Input: part model. Units: mm. Frame: model coordinates. A direction names the side the tool comes from. Round coordinates to 2 decimals unless told otherwise and drop trailing zeros. Write each loop counter-clockwise with the first axis right and the second up, starting at its lowest first coordinate (ties: lowest second). Pieces come first, ordered by that corner, then holes. Notation, with made-up numbers: (-9.75, 42.25) - (-3.75, 42.25) arc R38 ccw to (-3.75, 81.25) - close; hole circle Ø1 at (57, -30.5). An arc over 180 degrees is marked (long way). Use one line per item in the form item = value.
```python
from build123d import *

# Parameters (mm, degrees)
SKETCH1_R           = 2.25
SKETCH1_R_2         = 1.5
BOSS_EXTRUDE1_DEPTH = 1


with BuildPart() as part:
    # Sketch1 → Boss-Extrude1 (new body)
    with BuildSketch(Plane.XY):
        with BuildLine():
            Line((20, 42.5), (20, 47.75))
            ThreePointArc((20, 47.75), (19.414213562, 49.164213562), (18, 49.75))
            Line((18, 49.75), (-10, 49.75))
            ThreePointArc((-10, 49.75), (-10.71364418, 49.618344718), (-11.333333333, 49.240711985))
            ThreePointArc((-11.333333333, 49.240711985), (-12, 48.986067977), (-12.666666667, 49.240711985))
            ThreePointArc((-12.666666667, 49.240711985), (-13.28635582, 49.618344718), (-14, 49.75))
            Line((-14, 49.75), (-40, 49.75))
            ThreePointArc((-40, 49.75), (-40.71364418, 49.618344718), (-41.333333333, 49.240711985))
            ThreePointArc((-41.333333333, 49.240711985), (-42, 48.986067977), (-42.666666667, 49.240711985))
            ThreePointArc((-42.666666667, 49.240711985), (-43.28635582, 49.618344718), (-44, 49.75))
            Line((-44, 49.75), (-72, 49.75))
            ThreePointArc((-72, 49.75), (-73.414213562, 49.164213562), (-74, 47.75))
            Line((-74, 47.75), (-74, -7.25))
            ThreePointArc((-74, -7.25), (-73.414213562, -8.664213562), (-72, -9.25))
            Line((-72, -9.25), (-44, -9.25))
            ThreePointArc((-44, -9.25), (-43.28635582, -9.118344718), (-42.666666667, -8.740711985))
            ThreePointArc((-42.666666667, -8.740711985), (-42, -8.486067977), (-41.333333333, -8.740711985))
            ThreePointArc((-41.333333333, -8.740711985), (-40.71364418, -9.118344718), (-40, -9.25))
            Line((-40, -9.25), (-14, -9.25))
            ThreePointArc((-14, -9.25), (-13.28635582, -9.118344718), (-12.666666667, -8.740711985))
            ThreePointArc((-12.666666667, -8.740711985), (-12, -8.486067977), (-11.333333333, -8.740711985))
            ThreePointArc((-11.333333333, -8.740711985), (-10.71364418, -9.118344718), (-10, -9.25))
            Line((-10, -9.25), (18, -9.25))
            ThreePointArc((18, -9.25), (19.414213562, -8.664213562), (20, -7.25))
            Line((20, -7.25), (20, -2))
            ThreePointArc((20, -2), (19.414213562, -0.585786438), (18, 0))
            Line((18, 0), (0, 0))
            Line((0, 0), (0, 40.5))
            Line((0, 40.5), (18, 40.5))
            ThreePointArc((18, 40.5), (19.414213562, 41.085786438), (20, 42.5))
        make_face()
        with Locations((5.25, 44.75)):
            Circle(SKETCH1_R, mode=Mode.SUBTRACT)
        with Locations((14.75, 44.75)):
            Circle(SKETCH1_R, mode=Mode.SUBTRACT)
        with Locations((14.75, -4.25)):
            Circle(SKETCH1_R, mode=Mode.SUBTRACT)
        with Locations((5.25, -4.25)):
            Circle(SKETCH1_R, mode=Mode.SUBTRACT)
        with Locations((-27, 39.75)):
            Circle(SKETCH1_R, mode=Mode.SUBTRACT)
        with Locations((-27, 29.75)):
            Circle(SKETCH1_R, mode=Mode.SUBTRACT)
        with Locations((-27, 19.75)):
            Circle(SKETCH1_R, mode=Mode.SUBTRACT)
        with Locations((-27, 9.749358603)):
            Circle(SKETCH1_R, mode=Mode.SUBTRACT)
        with Locations((-27, -0.250641397)):
            Circle(SKETCH1_R, mode=Mode.SUBTRACT)
        with Locations((-64, 10.14)):
            Circle(SKETCH1_R_2, mode=Mode.SUBTRACT)
    extrude(amount=BOSS_EXTRUDE1_DEPTH)


solid = part.part
```
(1) Cut plane D-D on x = -64. Output: boundary loops of the cut face in (y, z).
Derived:
outline = (-9.25, 0) - (8.64, 0) - (8.64, 1) - (-9.25, 1) - close; (11.64, 0) - (49.75, 0) - (49.75, 1) - (11.64, 1) - close
(2) Cut plane A-A on x = 5.25. Output: boundary loops of the cut face in (y, z), then the cut area to 3 significant figures.
Derived:
outline = (-9.25, 0) - (-6.5, 0) - (-6.5, 1) - (-9.25, 1) - close; (-2, 0) - (0, 0) - (0, 1) - (-2, 1) - close; (40.5, 0) - (42.5, 0) - (42.5, 1) - (40.5, 1) - close; (47, 0) - (49.75, 0) - (49.75, 1) - (47, 1) - close
area = 9.50 mm^2
(3) Cut plane B-B on x = -27. Output: boundary loops of the cut face in (y, z), then the cut area to 3 significant figures.
Derived:
outline = (-9.25, 0) - (-2.5, 0) - (-2.5, 1) - (-9.25, 1) - close; (2, 0) - (7.5, 0) - (7.5, 1) - (2, 1) - close; (12, 0) - (17.5, 0) - (17.5, 1) - (12, 1) - close; (22, 0) - (27.5, 0) - (27.5, 1) - (22, 1) - close; (32, 0) - (37.5, 0) - (37.5, 1) - (32, 1) - close; (42, 0) - (49.75, 0) - (49.75, 1) - (42, 1) - close
area = 36.5 mm^2
(4) Material intervals for L1, parallel to Y at x = 5.25, z = 0.45; L2, parallel to Y at x = -27, z = 0.3; L3, parallel to X at y = 11, z = 0.75, sorted ascending.
Derived:
L1 = -9.25 to -6.5, -2 to 0, 40.5 to 42.5, 47 to 49.75
L2 = -9.25 to -2.5, 2 to 7.5, 12 to 17.5, 22 to 27.5, 32 to 37.5, 42 to 49.75
L3 = -74 to -65.23, -62.77 to -28.87, -25.13 to 0
(5) Draft query along X for faces 3 (the face through (-38, 21, 1)), 4 (the face through (-73.4, 49.18, 0.49)), 5 (the face through (7.396, -3.574, 0.493)), 6 (the face through (-25.962, 7.753, 0.493)). Return one class per face: released by +X, released by -X, zero draft, split by the parting line, or undercut.
Derived:
face_3 = zero draft
face_4 = released by -X
face_5 = undercut
face_6 = undercut
(6) Access query for faces 1 (the face through (19.43, 49.15, 0.49)), 2 (the face through (19.4, 41.07, 0.49)). Directions: +Z, -Z, +X, -X, +Y, -Y. A direction counts if a zero-diameter tool reaches every point of the face in a straight line with its end or side. Return the directions, or none.
Derived:
face_1 = +Z, -Z, +X, +Y
face_2 = +Z, -Z, +X
(7) Cut plane C-C on y = -4.25. Output: boundary loops of the cut face in (x, z).
Derived:
outline = (-74, 0) - (3, 0) - (3, 1) - (-74, 1) - close; (7.5, 0) - (12.5, 0) - (12.5, 1) - (7.5, 1) - close; (17, 0) - (20, 0) - (20, 1) - (17, 1) - close
